from build123d import *

# Parameters (mm, degrees)
SKETCH1_R              = 1.75
BASE_SHAPE_DEPTH       = 8.2
SKETCH3_W              = 2
SKETCH3_H              = 20.5
STRAP_CUT_DEPTH        = 53.32064602
XT60_CUT_REACH         = 70.811
SKETCH5_R              = 1
POWER_WIRES_CUT_DEPTH  = 53.32064602
SKETCH6_W              = 23.7
SKETCH6_H              = 5
IO_WIRES_CUT_DEPTH     = 6
BOTTOM_DEPTH           = 36
BOTTOM_START           = -1
BOTTOM_HOLES_OUTLINE_R = 1.75
BOTTOM_HOLES_DEPTH     = 1
SKETCH8_W              = 36.5
SKETCH8_H              = 46.5
PCB_CUT_DEPTH          = 1.7
LEDBAR_WIRES_CUT_REACH = 73.411
SKETCH13_W             = 3.2
SKETCH13_H             = 8.2
LEDBAR_SIDES_DEPTH     = 1.6
SKETCH14_R             = 0.95
LEDBAR_MOUNTS_DEPTH    = 2
SKETCH16_W             = 13.75
SKETCH16_H             = 4.15
SKETCH16_W_2           = 1.3
SKETCH16_H_2           = 1.2
BALANCE_PLUG_CUT_DEPTH = 6


with BuildPart() as part:
    # Sketch1 → Base shape (new body)
    with BuildSketch(Plane.XY):
        with BuildLine():
            ThreePointArc((-15.5, 31.1), (-18.328427125, 29.928427125), (-19.5, 27.1))
            Line((-19.5, 27.1), (-19.5, -32.6))
            Line((-19.5, -32.6), (19.5, -32.6))
            Line((19.5, -32.6), (19.5, 21.2))
            Line((19.5, 21.2), (24.7, 26.4))
            Line((24.7, 26.4), (24.7, 33.9))
            Line((24.7, 33.9), (7.95, 33.9))
            Line((7.95, 33.9), (7.95, 31.1))
            Line((7.95, 31.1), (-15.5, 31.1))
        make_face()
        with Locations((-15.25, -23.35)):
            Circle(SKETCH1_R, mode=Mode.SUBTRACT)
        with Locations((15.25, -23.35)):
            Circle(SKETCH1_R, mode=Mode.SUBTRACT)
        with BuildLine():
            Line((-18, -20.35), (-18, 4.15))
            Line((-18, 4.15), (-15.25, 4.15))
            ThreePointArc((-15.25, 4.15), (-12.25, 7.15), (-15.25, 10.15))
            Line((-15.25, 10.15), (-18, 10.15))
            Line((-18, 10.15), (-18, 14.9))
            Line((-18, 14.9), (18, 14.9))
            Line((18, 14.9), (18, 10.15))
            Line((18, 10.15), (15.25, 10.15))
            ThreePointArc((15.25, 10.15), (12.25, 7.15), (15.25, 4.15))
            Line((15.25, 4.15), (18, 4.15))
            Line((18, 4.15), (18, -20.35))
            Line((18, -20.35), (15.25, -20.35))
            ThreePointArc((15.25, -20.35), (12.25, -23.35), (15.25, -26.35))
            Line((15.25, -26.35), (18, -26.35))
            Line((18, -26.35), (18, -31.1))
            Line((18, -31.1), (-18, -31.1))
            Line((-18, -31.1), (-18, -26.35))
            Line((-18, -26.35), (-15.25, -26.35))
            ThreePointArc((-15.25, -26.35), (-12.25, -23.35), (-15.25, -20.35))
            Line((-15.25, -20.35), (-18, -20.35))
        make_face(mode=Mode.SUBTRACT)
        with Locations((-15.25, 7.15)):
            Circle(SKETCH1_R, mode=Mode.SUBTRACT)
        with Locations((-15.25, 25.15)):
            Circle(SKETCH1_R, mode=Mode.SUBTRACT)
        with Locations((15.25, 7.15)):
            Circle(SKETCH1_R, mode=Mode.SUBTRACT)
        with Locations((15.25, 25.15)):
            Circle(SKETCH1_R, mode=Mode.SUBTRACT)
    extrude(amount=BASE_SHAPE_DEPTH)

    # Sketch3 → Strap cut (cut, through all)
    with BuildSketch(Plane(origin=(19.5, 0, 0), x_dir=(0, 0, -1), z_dir=(1, 0, 0))):
        with Locations((-1, -8.1)):
            Rectangle(SKETCH3_W, SKETCH3_H)
    extrude(amount=-STRAP_CUT_DEPTH, mode=Mode.SUBTRACT)

    # Sketch4 → XT60 cut (cut, up to next)
    with BuildSketch(Plane(origin=(0, 31.1, 0), x_dir=(1, 0, 0), z_dir=(0, 1, 0)), mode=Mode.PRIVATE) as xt60_cut_sk1:
        Polygon((7.95, -8.2), (7.95, 0), (-5.099802631, 0), (-7.95, -2.555349365), (-7.95, -5.644650635), (-5.099802631, -8.2), align=None)
    xt60_cut_tool1 = extrude(xt60_cut_sk1.sketch, amount=-XT60_CUT_REACH, mode=Mode.PRIVATE) & part.part
    add(xt60_cut_tool1.solids().sort_by_distance((0.414164, 31.1, 4.1))[0], mode=Mode.SUBTRACT)

    # Sketch5 → Power wires cut (cut, through all)
    with BuildSketch(Plane(origin=(19.5, 0, 0), x_dir=(0, 0, -1), z_dir=(1, 0, 0))):
        with Locations((-5.2, 13.9)):
            Circle(SKETCH5_R)
        with Locations((-5.2, 11.9)):
            Circle(SKETCH5_R)
        with BuildLine():
            ThreePointArc((-5.2, 12.9), (-5.907106781, 13.192893219), (-6.2, 13.9))
            Line((-6.2, 13.9), (-6.2, 11.9))
            ThreePointArc((-6.2, 11.9), (-5.907106781, 12.607106781), (-5.2, 12.9))
        make_face()
        with BuildLine():
            Line((-4.2, 11.9), (-4.2, 13.9))
            ThreePointArc((-4.2, 13.9), (-4.492893219, 13.192893219), (-5.2, 12.9))
            ThreePointArc((-5.2, 12.9), (-4.492893219, 12.607106781), (-4.2, 11.9))
        make_face()
        with Locations((-5.2, -30.1)):
            Circle(SKETCH5_R)
        with Locations((-5.2, -28.1)):
            Circle(SKETCH5_R)
        with BuildLine():
            ThreePointArc((-5.2, -29.1), (-4.492893219, -29.392893219), (-4.2, -30.1))
            Line((-4.2, -30.1), (-4.2, -28.1))
            ThreePointArc((-4.2, -28.1), (-4.492893219, -28.807106781), (-5.2, -29.1))
        make_face()
        with BuildLine():
            Line((-6.2, -28.1), (-6.2, -30.1))
            ThreePointArc((-6.2, -30.1), (-5.907106781, -29.392893219), (-5.2, -29.1))
            ThreePointArc((-5.2, -29.1), (-5.907106781, -28.807106781), (-6.2, -28.1))
        make_face()
    extrude(amount=-POWER_WIRES_CUT_DEPTH, mode=Mode.SUBTRACT)

    # Sketch6 → IO wires cut (cut)
    with BuildSketch(Plane.XY.offset(8.2)):
        with BuildLine():
            ThreePointArc((-10.85, 20.9), (-11.557106781, 20.607106781), (-11.85, 19.9))
            Line((-11.85, 19.9), (11.85, 19.9))
            ThreePointArc((11.85, 19.9), (11.557106781, 20.607106781), (10.85, 20.9))
            Line((10.85, 20.9), (-10.85, 20.9))
        make_face()
        with Locations((0, 17.4)):
            Rectangle(SKETCH6_W, SKETCH6_H)
    extrude(amount=-IO_WIRES_CUT_DEPTH, mode=Mode.SUBTRACT)

    # Bottom: read off the stored shape, not the designer's step
    # Bottom outline → Bottom (add)
    with BuildSketch(Plane(origin=(-18, 0, 0), x_dir=(0, 0, -1), z_dir=(1, 0, 0))):
        Polygon((0, -18.35), (-2, -18.35), (-2, 2.15), (0, 2.15), (0, 14.9), (-1, 14.9), (-1, 3.15), (-3, 3.15), (-3, -19.35), (-1, -19.35), (-1, -31.1), (0, -31.1), align=None)
    extrude(amount=BOTTOM_DEPTH)

    # Bottom holes: read off the stored shape, not the designer's step
    # Bottom holes outline → Bottom holes (cut)
    with BuildSketch(Plane(origin=(0, 0, 0), x_dir=(-1, 0, 0), z_dir=(0, 0, -1)).offset(BOTTOM_START)):
        with Locations((-15.25, -23.35)):
            Circle(BOTTOM_HOLES_OUTLINE_R)
        with Locations((15.25, -23.35)):
            Circle(BOTTOM_HOLES_OUTLINE_R)
        with Locations((15.25, 7.15)):
            Circle(BOTTOM_HOLES_OUTLINE_R)
        with Locations((-15.25, 7.15)):
            Circle(BOTTOM_HOLES_OUTLINE_R)
    extrude(amount=BOTTOM_HOLES_DEPTH, mode=Mode.SUBTRACT)

    # Sketch8 → PCB cut (cut)
    with BuildSketch(Plane.XY.offset(8.2)):
        with Locations((0, -8.1)):
            Rectangle(SKETCH8_W, SKETCH8_H)
    extrude(amount=-PCB_CUT_DEPTH, mode=Mode.SUBTRACT)

    # Sketch11 → Ledbar wires cut (cut, up to next)
    with BuildSketch(Plane.XZ.offset(32.6), mode=Mode.PRIVATE) as ledbar_wires_cut_sk1:
        with BuildLine():
            Line((-2.5, 4.45), (2.5, 4.45))
            ThreePointArc((2.5, 4.45), (3.207106781, 4.157106781), (3.5, 3.45))
            Line((3.5, 3.45), (3.5, 2.95))
            ThreePointArc((3.5, 2.95), (3.207106781, 2.242893219), (2.5, 1.95))
            Line((2.5, 1.95), (-2.5, 1.95))
            ThreePointArc((-2.5, 1.95), (-3.207106781, 2.242893219), (-3.5, 2.95))
            Line((-3.5, 2.95), (-3.5, 3.45))
            ThreePointArc((-3.5, 3.45), (-3.207106781, 4.157106781), (-2.5, 4.45))
        make_face()
    ledbar_wires_cut_tool1 = extrude(ledbar_wires_cut_sk1.sketch, amount=-LEDBAR_WIRES_CUT_REACH, mode=Mode.PRIVATE) & part.part
    add(ledbar_wires_cut_tool1.solids().sort_by_distance((0, -32.6, 3.2))[0], mode=Mode.SUBTRACT)

    # Sketch13 → Ledbar sides (add)
    with BuildSketch(Plane.XZ.offset(32.6)):
        with Locations((17.9, 4.1)):
            Rectangle(SKETCH13_W, SKETCH13_H)
        with Locations((-17.9, 4.1)):
            Rectangle(SKETCH13_W, SKETCH13_H)
    extrude(amount=LEDBAR_SIDES_DEPTH)

    # Sketch14 → Ledbar mounts (add)
    with BuildSketch(Plane.XZ.offset(32.6)):
        with Locations(Location((8, 6.85, 0), (0, 0, 180))):
            Circle(SKETCH14_R)
        with Locations(Location((-8, 6.85, 0), (0, 0, 180))):
            Circle(SKETCH14_R)
    extrude(amount=LEDBAR_MOUNTS_DEPTH)

    # Sketch16 → Balance plug cut (cut)
    with BuildSketch(Plane(origin=(0, 33.9, 0), x_dir=(1, 0, 0), z_dir=(0, 1, 0))):
        with Locations((16.325, -6.125)):
            Rectangle(SKETCH16_W, SKETCH16_H)
        with Locations((11.625, -3.45)):
            Rectangle(SKETCH16_W_2, SKETCH16_H_2)
        with Locations((21.025, -3.45)):
            Rectangle(SKETCH16_W_2, SKETCH16_H_2)
    extrude(amount=-BALANCE_PLUG_CUT_DEPTH, mode=Mode.SUBTRACT)


solid = part.part
Design review of the part built by this model. Coordinates are the model's own, in mm. A direction names the side the tool comes from. Coordinates: 2 decimals unless noted, no trailing zeros. Write each loop counter-clockwise with the first axis right and the second up, starting at its lowest first coordinate (ties: lowest second). Pieces come first, ordered by that corner, then holes. Notation, with made-up numbers: (19, 75) -> (49, 75) arc R12 cw to (49, 89) -> close; hole circle Ø7 at (8.25, -31.5). An arc over 180 degrees is marked (long way). Write each question's results on one line, items separated by ' | '. Start each with the question number.
(1) The part is to be moulded in two halves that separate along X. For faces 6 (the face through (9.45, 31, 6)), 7 (the face through (0, -8, 2)), say which applies: pulls with the +X half, pulls with the -X half, needs draft (parallel to the pull), parting line crosses it, or undercut.
(2) Clearance check with flat-ended pins moving along their axes: P1, Ø3.5, axis at x = 4.5, y = -27.5, coming from the +Z side; P2, Ø3, axis at x = -16, z = 4, coming from the -Y side; P3, Ø1.4, axis at x = 17.5, z = 5, coming from the +Y side. State where each tip first meets the part, or that it passes through.
(3) Take a section at B-B on x = 0.5. Write out the cut boundary in (y, z).
(4) Tool access review of faces 1 (the face through (21, 31, 2.85)), 2 (the face through (19, -29, 6.2)), 3 (the face through (-18.25, -8, 7)), 4 (the face through (-6.505, 23.113, 1.26)), 5 (the face through (0, 2.15, 1)): name each direction out of +Z, -Z, +X, -X, +Y, -Y from which nothing blocks a thin tool from reaching the whole face with its end or side.
(5) Take a section at A-A on y = 7.15. Write out the cut boundary in (x, z).
(6) For line 1 along X through (y, z) = (-23.35, 3.5); line 2 along Y through (x, z) = (-6.5, 1.5); line 3 along X through (y, z) = (-13, 7.5), list the stretches that pass through material, from the lowest coordinate up. Write a range as from..to.
(7) Take a section at D-D on y = -5.5. Write out the cut boundary in (x, z), and give its area (4 significant figures).
(8) Take a section at C-C on y = 25.15. Write out the cut boundary in (x, z).
Results found:
1) face 6: undercut | face 7: needs draft
2) P1: stops at z = 1 | P2: stops at y = -34.2 | P3: stops at y = 27.9
3) outline: (-32.6, 0) -> (-18.35, 0) -> (-18.35, 2) -> (2.15, 2) -> (2.15, 0) -> (14.9, 0) -> (14.9, 1) -> (3.15, 1) -> (3.15, 3) -> (-19.35, 3) -> (-19.35, 1) -> (-31.1, 1) -> (-31.1, 1.95) -> (-32.6, 1.95) -> close; (-32.6, 4.45) -> (-31.1, 4.45) -> (-31.1, 6.5) -> (-31.35, 6.5) -> (-31.35, 8.2) -> (-32.6, 8.2) -> close
4) face 1: +Z, +Y | face 2: +X, -X | face 3: +Z | face 4: +Y | face 5: -Z, +X, -X
5) outline: (-19.5, 0) -> (-17, 0) -> (-17, 6.5) -> (-18.25, 6.5) -> (-18.25, 8.2) -> (-19.5, 8.2) -> close; (-13.5, 0) -> (13.5, 0) -> (13.5, 6.5) -> (12.25, 6.5) -> (12.25, 1) -> (-12.25, 1) -> (-12.25, 6.5) -> (-13.5, 6.5) -> close; (17, 0) -> (19.5, 0) -> (19.5, 8.2) -> (18.25, 8.2) -> (18.25, 6.5) -> (17, 6.5) -> close
6) line 1: x = -19.5..-17, -13.5..-12.25, 12.25..13.5, 17..19.5 | line 2: y = -32.6..-31.1, -19.35..-18.35, 2.15..3.15 | line 3: x = -19.5..-18.25, 18.25..19.5
7) outline: (-19.5, 2) -> (19.5, 2) -> (19.5, 8.2) -> (18.25, 8.2) -> (18.25, 6.5) -> (18, 6.5) -> (18, 3) -> (-18, 3) -> (-18, 6.5) -> (-18.25, 6.5) -> (-18.25, 8.2) -> (-19.5, 8.2) -> close | area: 53.75 mm2
8) outline: (-19.5, 0) -> (-17, 0) -> (-17, 8.2) -> (-19.5, 8.2) -> close; (-13.5, 0) -> (-5.1, 0) -> (-7.95, 2.56) -> (-7.95, 5.64) -> (-5.1, 8.2) -> (-13.5, 8.2) -> close; (7.95, 0) -> (13.5, 0) -> (13.5, 8.2) -> (7.95, 8.2) -> close; (17, 0) -> (23.45, 0) -> (23.45, 8.2) -> (17, 8.2) -> close
